from build123d import *

# Parameters (mm, degrees)
F1_R     = 2.75
F1_R_2   = 1.5
F2_DEPTH = 2
F3_START = 1.5
F3_DEPTH = 0.5
F4_START = 2
F4_DEPTH = 36
F5_SIZE2 = 1.25
F5_SIZE  = 1.25
F6_R     = 0.25


# Not quite as in the source:
# - a feature names something its author has since deleted; it is built from what else it names


with BuildPart() as f2:
    # F1 (on Top) → F2 (new body)
    with BuildSketch(Plane.XY):
        Circle(F1_R)
        Circle(F1_R_2, mode=Mode.SUBTRACT)
        Circle(F1_R_2)
        Polygon((-0.5773502692, -1), (-1.1547005384, 0), (-0.5773502692, 1), (0.5773502692, 1), (1.1547005384, 0), (0.5773502692, -1), align=None, mode=Mode.SUBTRACT)
    extrude(amount=F2_DEPTH)

    # F1 (on Top) → F3 (join)
    with BuildSketch(Plane.XY.offset(F3_START)):
        Polygon((-0.5773502692, 1), (-1.1547005384, 0), (-0.5773502692, -1), (0.5773502692, -1), (1.1547005384, 0), (0.5773502692, 1), align=None)
    extrude(amount=F3_DEPTH)

    # F1 (on Top) → F4 (join)
    with BuildSketch(Plane.XY.offset(F4_START)):
        Circle(F1_R_2)
        Polygon((-0.5773502692, -1), (-1.1547005384, 0), (-0.5773502692, 1), (0.5773502692, 1), (1.1547005384, 0), (0.5773502692, -1), align=None, mode=Mode.SUBTRACT)
        Polygon((-0.5773502692, 1), (-1.1547005384, 0), (-0.5773502692, -1), (0.5773502692, -1), (1.1547005384, 0), (0.5773502692, 1), align=None)
    extrude(amount=F4_DEPTH)

    # F5
    f5_edges = [f2.edges().sort_by_distance(p)[0] for p in [
        (-2.75, 0, 0),
    ]]
    chamfer(f5_edges, length=F5_SIZE, length2=F5_SIZE2)

    # F6
    f6_edges = [f2.edges().sort_by_distance(p)[0] for p in [
        (-2.75, 0, 2),
        (-1.5, 0, 2),
        (-1.5, 0, 0),
        (-2.75, 0, 1.25),
    ]]
    fillet(f6_edges, radius=F6_R)


solid = f2.part
Input: part model. Units: mm. Frame: model coordinates. A direction names the side the tool comes from. Round coordinates to 2 decimals unless told otherwise and drop trailing zeros. Loops run counter-clockwise (first coordinate to the right, second up) from the corner with the lowest first, then second, coordinate; pieces in that order, holes last. Notation, with made-up numbers: (-21, -29.5) -> (-2, -29.5) arc R14 cw to (-2, -11.5) -> close; hole circle Ø8 at (53, 34.25). An arc over 180 degrees is marked (long way). Answer as a JSON object with one key per item and string values. Group by question number.
1) Section query A-A on z = 14. Output: boundary loops of the cut face in (x, y), plus the area to 3 significant figures.
2) Draft query along X for faces 1 (the cylindrical face through (-1.5, 0.07, 19.87)), 2 (the flat face through (0, -1, 1)), 3 (the flat face through (0, 0, 38)). Return one class per face: +X half, -X half, draft (parallel to the pull), parting line (faces both ways), or undercut.
3) Pin query (flat end, axial travel): pin 1 (1 mm diameter, centred on x = 1.5, z = 19, fed in from -Y); pin 2 (0.9 mm diameter, centred on x = 0, z = 0.5, fed in from +Y); pin 3 (0.6 mm diameter, centred on x = 0, z = 1, fed in from -Y). Return the tip coordinate at first contact, or that it passes through.
4) Ray query, L1, parallel to Z at x = 0.5, y = -0.55; L2, parallel to Z at x = 1.45, y = 0; L3, parallel to Y at x = 0.05, z = 12. Return the intervals inside material, ascending.
5) Reachability of faces 4 (the flat face through (-0.87, 0.49, 0.74)), 5 (the flat face through (1, 2, 2)), 6 (the cylindrical face through (-0.596, -2.685, 1.549)) from +Z, -Z, +X, -X, +Y, -Y: full face, straight path, thin tool, end or side. Return the list, or none.
Reply:
{
 "1": {"outline": "circle Ø3 at (0, 0)", "area": "7.07 mm2"},
 "2": {"face 1": "parting line", "face 2": "undercut", "face 3": "draft"},
 "3": {"pin 1": "stops at y = -1.12", "pin 2": "stops at y = 2.45", "pin 3": "stops at y = -2.74"},
 "4": {"L1": "z = 1.5 to 38", "L2": "z = 0.01 to 38", "L3": "y = -1.5 to 1.5"},
 "5": {"face 4": "-Z", "face 5": "+Z", "face 6": "+Z, -Z"}
}
